from build123d import *

# Parameters (mm, degrees)
SKETCH1_W                 = 60.3123
SKETCH1_H                 = 19.05
EXTRUDE1_DEPTH            = 6.35
SKETCH2_R                 = 1.778
CUT_EXTRUDE1_DEPTH        = 7.35
F_6_32_TAPPED_HOLE1_D     = 2.7051
F_6_32_TAPPED_HOLE1_DEPTH = 9.525
F_6_32_TAPPED_HOLE1_TIP   = 0.81269403
F_6_32_TAPPED_HOLE2_D     = 2.7051
F_6_32_TAPPED_HOLE2_DEPTH = 9.525
F_6_32_TAPPED_HOLE2_TIP   = 0.81269403


with BuildPart() as part:
    # Sketch1 → Extrude1 (new body)
    with BuildSketch(Plane.XY):
        with Locations((30.15615, 9.525)):
            Rectangle(SKETCH1_W, SKETCH1_H)
    extrude(amount=EXTRUDE1_DEPTH)

    # Sketch2 → Cut-Extrude1 (cut, through all)
    with BuildSketch(Plane.XY.offset(6.35)):
        with Locations((9.525, 9.525)):
            Circle(SKETCH2_R)
        with Locations((50.7873, 9.525)):
            Circle(SKETCH2_R)
    extrude(amount=-CUT_EXTRUDE1_DEPTH, mode=Mode.SUBTRACT)

    # #6-32 Tapped Hole1
    with Locations(Plane.ZY):
        with Locations((3.175, 9.525)):
            Hole(F_6_32_TAPPED_HOLE1_D / 2, depth=F_6_32_TAPPED_HOLE1_DEPTH)
            with Locations((0, 0, -(F_6_32_TAPPED_HOLE1_DEPTH + F_6_32_TAPPED_HOLE1_TIP / 2))):  # 118° drill point
                Cone(0, F_6_32_TAPPED_HOLE1_D / 2, F_6_32_TAPPED_HOLE1_TIP, mode=Mode.SUBTRACT)

    # #6-32 Tapped Hole2
    with Locations(Plane(origin=(60.3123, 0, 0), x_dir=(0, 0, -1), z_dir=(1, 0, 0))):
        with Locations((-3.175, 9.525)):
            Hole(F_6_32_TAPPED_HOLE2_D / 2, depth=F_6_32_TAPPED_HOLE2_DEPTH)
            with Locations((0, 0, -(F_6_32_TAPPED_HOLE2_DEPTH + F_6_32_TAPPED_HOLE2_TIP / 2))):  # 118° drill point
                Cone(0, F_6_32_TAPPED_HOLE2_D / 2, F_6_32_TAPPED_HOLE2_TIP, mode=Mode.SUBTRACT)


solid = part.part
For this review, take the finished solid that the model builds, in its own axes (mm). A direction names the side the tool comes from. Round coordinates to 2 decimals unless told otherwise and drop trailing zeros. Write each loop counter-clockwise with the first axis right and the second up, starting at its lowest first coordinate (ties: lowest second). Pieces come first, ordered by that corner, then holes. Notation, with made-up numbers: (-33.5, 62.25) -> (19.5, 62.25) arc R26 ccw to (19.5, 85.25) -> close; hole circle Ø6 at (-12.75, 89). An arc over 180 degrees is marked (long way). Use CSV: the item, a comma, the result in double quotes.
(1) For faces 1 (the face through (30, 10, 6.35)), 2 (the face through (56.068, 10.866, 2.999)), list the 3-axis set-ups (+Z, -Z, +X, -X, +Y, -Y) from which the entire face can be reached by the end or side of a thin tool; tool diameter is ignored.
Computed values:
face 1,"+Z, +X, -X, +Y, -Y"
face 2,"+X"
(2) Consider section C-C, the plane x = 4. Give the boundary of the cut face in (y, z) (3 decimals).
Computed values:
outline,"(0, 0) -> (19.05, 0) -> (19.05, 6.35) -> (0, 6.35) -> close; hole circle Ø2.705 at (9.525, 3.175)"
(3) To check wall thickness, follow L1, parallel to X at y = 11, z = 2; L2, parallel to X at y = 8, z = 1.5; L3, parallel to Y at x = 51, z = 2.25. State the ranges of each line that lie inside material, in increasing order. Write a range as [from, to].
Computed values:
L1,"[0, 8.53], [10.52, 49.79], [51.78, 60.31]"
L2,"[0, 8.61], [10.44, 49.87], [51.7, 60.31]"
L3,"[0, 7.76], [11.29, 19.05]"
(4) Clearance check with a flat-ended pin moving along its axis: P1, Ø5.5, axis at x = 9.525, y = 9.525, coming from the +Z side. State where the tip first meets the part, or that it passes through.
Computed values:
P1,"z = 6.35"
(5) Consider section B-B, the plane z = 3.5. Give the boundary of the cut face in (x, y) (3 decimals).
Computed values:
outline,"(0, 0) -> (60.312, 0) -> (60.312, 8.212) -> (51.986, 8.212) arc R1.778 cw (long way) to (51.986, 10.838) -> (60.312, 10.838) -> (60.312, 19.05) -> (0, 19.05) -> (0, 10.838) -> (8.326, 10.838) arc R1.778 cw (long way) to (8.326, 8.212) -> (0, 8.212) -> close"
(6) Draft analysis for pull direction Y (two halves, no side actions). For faces 3 (the face through (4.244, 10.866, 3.351)), 4 (the face through (30, 19.05, 3)), 5 (the face through (60.312, 9, 5)), state which applies: +Y half, -Y half, draft (parallel to the pull), parting line (faces both ways), or undercut.
Computed values:
face 3,"undercut"
face 4,"+Y half"
face 5,"draft"
(7) Consider section A-A, the plane z = 1.25. Give the boundary of the cut face in (x, y) (3 decimals).
Computed values:
outline,"(0, 0) -> (60.312, 0) -> (60.312, 19.05) -> (0, 19.05) -> close; hole circle Ø3.556 at (9.525, 9.525); hole circle Ø3.556 at (50.787, 9.525)"
